The listing builds one solid part. Answer for the finished solid, in the listing's coordinates (mm). Face numbers are marked on the shaded views. Give positions to 0.01 mm unless a question says otherwise; leave off trailing zeros. Loops run counter-clockwise (first coordinate to the right, second up) from the corner with the lowest first, then second, coordinate; pieces in that order, holes last. Notation, with made-up numbers: (6.25, 57) - (48.25, 57) arc R36 cw to (48.25, 96) - close; hole circle Ø8 at (40.5, -11.75). An arc over 180 degrees is marked (long way). Answer as CSV lines item,"result". Start each with the question number.
1) A cutting plane is placed at A-A (z = -24). Determine the outline of the cut face in (x, y).
2) A cutting plane is placed at D-D (x = 117.5). Determine the outline of the cut face in (y, z), and give its area (3 significant figures).
3) Flat-ended cylindrical pins translate along their axes: pin 1 (8 mm diameter, centred on y = 41.5, z = -127.5, fed in from +X); pin 2 (3 mm diameter, centred on x = 47, y = 29.5, fed in from +Z); pin 3 (8 mm diameter, centred on y = 7.5, z = -60, fed in from -X). Find the tip coordinate at first contact, or state that the pin passes through.
4) A cutting plane is placed at B-B (y = 31.5). Determine the outline of the cut face in (x, z), and give its area (3 significant figures).
5) A cutting plane is placed at C-C (x = 64). Determine the outline of the cut face in (y, z).
6) Find the intervals of material crossed by line 1 along X through (y, z) = (19.5, -95); line 2 along Y through (x, z) = (283.5, -29.5); line 3 along Z through (x, y) = (209, 54), in increasing order.
7) For a pull along Z with two mould halves and no side action, classify the marked faces 1, 2 and 3 as pulls with the +Z half, pulls with the -Z half, needs draft (parallel to the pull), parting line crosses it, or undercut.
```python
from build123d import *

# Parameters (mm, degrees)
BOSS_EXTRUDE1_DEPTH = 70
CUT_EXTRUDE1_DEPTH  = 402
CUT_EXTRUDE3_DEPTH  = 164
SKETCH5_R           = 22.231226606
CUT_EXTRUDE4_DEPTH  = 251


with BuildPart() as part:
    # Sketch1 → Boss-Extrude1 (new body)
    with BuildSketch(Plane(origin=(0, 0, 0), x_dir=(1, 0, 0), z_dir=(0, 1, 0))):
        Polygon((0, 0), (353.553390593, 0), (176.776695297, 176.776695297), align=None)
    extrude(amount=BOSS_EXTRUDE1_DEPTH)

    # Sketch3 → Cut-Extrude1 (cut)
    with BuildSketch(Plane(origin=(0, 0, 0), x_dir=(0, 0, -1), z_dir=(1, 0, 0))):
        with BuildLine():
            Line((0, 70), (0, 0))
            ThreePointArc((0, 0), (35, 35), (0, 70))
        make_face()
    extrude(amount=CUT_EXTRUDE1_DEPTH, mode=Mode.SUBTRACT)

    # Sketch4 → Cut-Extrude3 (cut)
    with BuildSketch(Plane.XZ):
        Polygon((318.553390593, -35), (283.553390593, 0), (353.553390593, 0), align=None)
    extrude(amount=-CUT_EXTRUDE3_DEPTH, mode=Mode.SUBTRACT)

    # Sketch5 → Cut-Extrude4 (cut)
    with BuildSketch(Plane(origin=(0, 0, 0), x_dir=(-0.7071067811865462, 0, 0.7071067811865489), z_dir=(-0.7071067811865489, 0, -0.7071067811865462))):
        with Locations((-195.507283553, 35)):
            Circle(SKETCH5_R)
    extrude(amount=-CUT_EXTRUDE4_DEPTH, mode=Mode.SUBTRACT)


solid = part.part
```
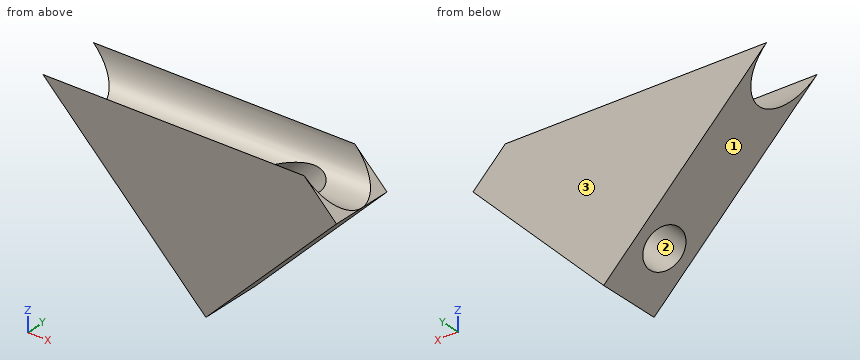
Ans:
1,outline,"(24, 0) - (307.55, 0) - (307.55, 9.52) - (24, 9.52) - close; (24, 60.48) - (307.55, 60.48) - (307.55, 70) - (24, 70) - close"
2,outline,"(0, -117.5) - (70, -117.5) - (70, 0) arc R35 cw to (0, 0) - close"
2,area,"6,300 mm2"
3,pin 1,"x = 230.05"
3,pin 2,"z = -34.29"
3,pin 3,"x = 56"
4,outline,"(34.82, -34.82) - (122.72, -122.72) - (210.62, -34.82) - close; (153.77, -153.77) - (176.78, -176.78) - (318.55, -35) - (318.38, -34.82) - (272.71, -34.82) - close"
4,area,"13,700 mm2"
5,outline,"(0, -64) - (70, -64) - (70, 0) arc R35 cw to (0, 0) - close"
6,line 1,"95 to 158.95, 204.03 to 258.55"
6,line 2,"0 to 16.17, 53.83 to 70"
6,line 3,"-144.55 to -83.81, -51.17 to -29.39"
7,face 1,"pulls with the -Z half"
7,face 2,"undercut"
7,face 3,"needs draft"
